Autodesk Inventor part; units mm, degrees
ref_plane "YZ Plane" through (0, 0, 0) normal (1, 0, 0) x (0, 1, 0)
ref_plane "XZ Plane" through (0, 0, 0) normal (0, 1, 0) x (-1, 0, 0)
ref_plane "XY Plane" through (0, 0, 0) normal (0, 0, 1) x (1, 0, 0)
sketch "Sketch1" plane through (0, 0, 0) normal (0, 0, 1) x (1, 0, 0)
  circle A0 centre (0, 0) radius 47.5
  circle A1 centre (0, 0) radius 33
  circle A2 centre (41.5, 0) radius 2.25
  circle A3 centre (29.3449, 29.3449) radius 2.25
  circle A4 centre (0, 41.5) radius 2.25
  circle A5 centre (-29.3449, 29.3449) radius 2.25
  circle A6 centre (-41.5, 0) radius 2.25
  circle A7 centre (-29.3449, -29.3449) radius 2.25
  circle A8 centre (0, -41.5) radius 2.25
  circle A9 centre (29.3449, -29.3449) radius 2.25
  dimension "d0" = 95
  dimension "d1" = 66
  dimension "d2" = 4.5
  dimension "d3" = 41.5
  dimension "d6" = 360
extrude "Extrusion1" add sketch "Sketch1" along normal blind 15
sketch "Sketch2" plane through (0, 0, 15) normal (0, 0, 1) x (1, 0, 0)
  circle A0 centre (41.5, 0) radius 2.25
  circle A1 centre (41.5, 0) radius 4
  circle A2 centre (29.3449, 29.3449) radius 4
  circle A3 centre (0, 41.5) radius 4
  circle A4 centre (-29.3449, 29.3449) radius 4
  circle A5 centre (-41.5, 0) radius 4
  circle A6 centre (-29.3449, -29.3449) radius 4
  circle A7 centre (0, -41.5) radius 4
  circle A8 centre (29.3449, -29.3449) radius 4
  point P0 (0, 0)
  dimension "d10" = 8
  dimension "d13" = 360
extrude "Extrusion2" cut sketch "Sketch2" against normal blind 4.65 contours A0 | A1 | A2 | A3 | A4 | A5 | A6 | A7 | A8
properties part number "Slewing A" material "Aluminum 6061"
Geometry: final body of the model. Coordinates: model frame, mm. A direction names the side the tool comes from. Round coordinates to 2 decimals unless told otherwise and drop trailing zeros. Order: outer loops, then holes, each group sorted by start corner. A loop starts at its lowest first (then second) coordinate and runs counter-clockwise, first axis right, second up. Notation, with made-up numbers: (3.5, 18.5) - (48.5, 18.5) arc R28 ccw to (48.5, 50.5) - close; hole circle Ø9 at (77, 10). An arc over 180 degrees is marked (long way). Use CSV: the item, a comma, the result in double quotes. Start each with the question number.
Q1. Section query C-C (x = -41.5). Return loops of the section in (y, z), and give its area (3 significant figures).
Q2. Access query for faces 5 (the face through (30.5, 12.6, 7.4)), 6 (the face through (43, -2, 10.35)). Directions: +Z, -Z, +X, -X, +Y, -Y. A direction counts if a zero-diameter tool reaches every point of the face in a straight line with its end or side. Return the directions, or none.
Q3. Mould query, pull axis X, two halves, no side actions, for faces 1 (the face through (-43.748, -0.099, 5.103)), 2 (the face through (-10.3, 46.37, 7.4)), 3 (the face through (-10.8, -31.4, 15)), 4 (the face through (-27.6, 27.6, 10.35)). Classes: +X half, -X half, draft (parallel to the pull), parting line (faces both ways), or undercut.
Q4. Section query D-D (z = 12.25). State how many separate pieces and enclosed holes the cut face has, and give its area (3 significant figures).
Q5. Material intervals for line 1 along Y through (x, z) = (0, 11.9); line 2 along Y through (x, z) = (0, 7.75); line 3 along X through (y, z) = (-28.5, 7.5), sorted ascending. Write a range as from..to.
Q6. Section query A-A (x = 0). Return loops of the section in (y, z), and give its area (3 significant figures).
Q7. First-contact query: pin 1 (2.5 mm diameter, centred on x = 40.5, y = 1, fed in from +Z); pin 2 (3.5 mm diameter, centred on x = 0, y = 41.5, fed in from -Z) (1 decimal); pin 3 (1.5 mm diameter, centred on x = -25, z = 8, fed in from +Y); pin 4 (2 mm diameter, centred on x = -19, z = 10.5, fed in from -Y). Flat tips, straight axial feed; report the tip coordinate or a pass-through.
Result set:
1,outline,"(-23.11, 0) - (-2.25, 0) - (-2.25, 10.35) - (-4, 10.35) - (-4, 15) - (-23.11, 15) - close; (2.25, 0) - (23.11, 0) - (23.11, 15) - (4, 15) - (4, 10.35) - (2.25, 10.35) - close"
1,area,"609 mm2"
2,face 5,"+Z, -Z"
2,face 6,"+Z"
3,face 1,"undercut"
3,face 2,"parting line"
3,face 3,"draft"
3,face 4,"undercut"
4,separate pieces,"1"
4,enclosed holes,"9"
4,area,"3,260 mm2"
5,line 1,"y = -47.5..-45.5, -37.5..-33, 33..37.5, 45.5..47.5"
5,line 2,"y = -47.5..-43.75, -39.25..-33, 33..39.25, 43.75..47.5"
5,line 3,"x = -38..-31.43, -27.26..-16.64, 16.64..27.26, 31.43..38"
6,outline,"(-47.5, 0) - (-43.75, 0) - (-43.75, 10.35) - (-45.5, 10.35) - (-45.5, 15) - (-47.5, 15) - close; (-39.25, 0) - (-33, 0) - (-33, 15) - (-37.5, 15) - (-37.5, 10.35) - (-39.25, 10.35) - close; (33, 0) - (39.25, 0) - (39.25, 10.35) - (37.5, 10.35) - (37.5, 15) - (33, 15) - close; (43.75, 0) - (47.5, 0) - (47.5, 15) - (45.5, 15) - (45.5, 10.35) - (43.75, 10.35) - close"
6,area,"267 mm2"
7,pin 1,"stops at z = 10.35"
7,pin 2,"passes through"
7,pin 3,"stops at y = 40.84"
7,pin 4,"stops at y = -43.96"
